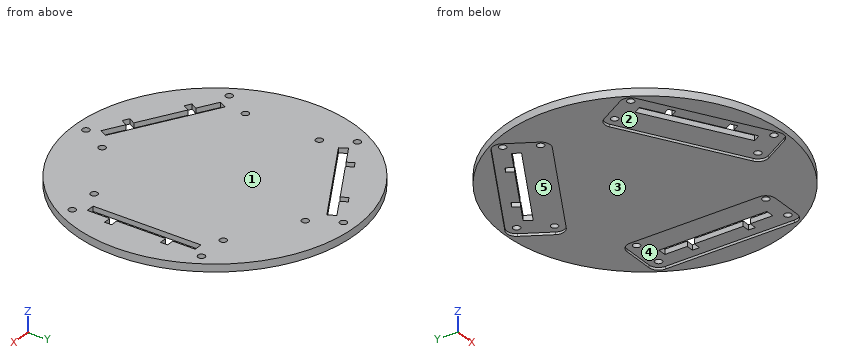
Autodesk Inventor part; units mm, degrees
ref_plane "YZ Plane" through (0, 0, 0) normal (1, 0, 0) x (0, 1, 0)
ref_plane "XZ Plane" through (0, 0, 0) normal (0, 1, 0) x (-1, 0, 0)
ref_plane "XY Plane" through (0, 0, 0) normal (0, 0, 1) x (1, 0, 0)
sketch "Skizze1" plane through (0, 0, 0) normal (0, 0, 1) x (1, 0, 0)
  line L0 (0, 78.2107) -> (0, -78.2107) construction
  line L1 (-128.6657, 0) -> (86.6199, 0) construction
  line L2 (31.7553, 29.05) -> (44.1553, 29.05) construction
  line L3 (47.5553, 25.65) -> (47.5553, -25.65) construction
  line L4 (44.1553, -29.05) -> (31.7553, -29.05) construction
  line L5 (28.3553, -25.65) -> (28.3553, 25.65) construction
  arc A0 (31.7553, 29.05) -> (28.3553, 25.65) centre (31.7553, 25.65) ccw construction
  arc A1 (47.5553, 25.65) -> (44.1553, 29.05) centre (44.1553, 25.65) ccw construction
  arc A2 (44.1553, -29.05) -> (47.5553, -25.65) centre (44.1553, -25.65) ccw construction
  arc A3 (28.3553, -25.65) -> (31.7553, -29.05) centre (31.7553, -25.65) ccw construction
  circle A4 centre (31.7553, 25.65) radius 1.4
  circle A5 centre (44.1553, 25.65) radius 1.4
  circle A6 centre (31.7553, -25.65) radius 1.4
  circle A7 centre (44.1553, -25.65) radius 1.4
  line L6 (41.6553, 21.4) -> (41.6553, -21.4)
  line L7 (38.3553, 21.4) -> (38.3553, -21.4)
  line L8 (38.3553, 21.4) -> (41.6553, 21.4)
  line L9 (38.3553, -21.4) -> (41.6553, -21.4)
  line L10 (38.3553, 0.8) -> (41.6553, 0.8)
  line L11 (38.3553, -0.8) -> (41.6553, -0.8)
  line L12 (41.6553, 12.5) -> (44.5713, 12.5)
  line L13 (44.5713, 12.5) -> (44.5713, 9.7)
  line L14 (44.5713, 9.7) -> (41.6553, 9.7)
  line L15 (41.6553, -9.7) -> (44.5713, -9.7)
  line L16 (44.5713, -9.7) -> (44.5713, -12.5)
  line L17 (44.5713, -12.5) -> (41.6553, -12.5)
  line L18 (44.1553, 29.45) -> (31.7553, 29.45)
  arc A8 (31.7553, 29.45) -> (27.9553, 25.65) centre (31.7553, 25.65) ccw
  line L19 (27.9553, 25.65) -> (27.9553, -25.65)
  arc A9 (27.9553, -25.65) -> (31.7553, -29.45) centre (31.7553, -25.65) ccw
  line L20 (31.7553, -29.45) -> (44.1553, -29.45)
  arc A10 (44.1553, -29.45) -> (47.9553, -25.65) centre (44.1553, -25.65) ccw
  line L21 (47.9553, -25.65) -> (47.9553, 25.65)
  arc A11 (47.9553, 25.65) -> (44.1553, 29.45) centre (44.1553, 25.65) ccw
  line L22 (25.9072, -29.1198) -> (28.4872, -27.589) construction
  line L23 (-0.6447, 43.9167) -> (-2.2947, 46.7745)
  circle A12 centre (0.1359, 51.0646) radius 1.4
  arc A13 (3.0804, 52.7646) -> (-1.5641, 54.0091) centre (0.1359, 51.0646) ccw construction
  arc A14 (3.4268, 52.9646) -> (-1.7641, 54.3555) centre (0.1359, 51.0646) ccw
  circle A15 centre (6.3359, 40.3259) radius 1.4
  line L24 (12.2649, 36.9962) -> (9.6492, 38.4652) construction
  arc A16 (8.0359, 37.3814) -> (9.2804, 42.0259) centre (6.3359, 40.3259) ccw construction
  arc A17 (8.2359, 37.035) -> (9.6268, 42.2259) centre (6.3359, 40.3259) ccw
  line L25 (9.6268, 42.2259) -> (3.4268, 52.9646)
  line L26 (3.0804, 52.7646) -> (9.2804, 42.0259) construction
  line L27 (-41.0357, 12.9759) -> (-47.2357, 23.7146) construction
  arc A18 (-41.0357, 12.9759) -> (-36.3912, 11.7314) centre (-38.0912, 14.6759) ccw construction
  circle A19 centre (-38.0912, 14.6759) radius 1.4
  circle A20 centre (-44.2912, 25.4146) radius 1.4
  arc A21 (-41.3821, 12.7759) -> (-36.1912, 11.385) centre (-38.0912, 14.6759) ccw
  line L28 (-47.5821, 23.5146) -> (-41.3821, 12.7759)
  arc A22 (-45.9912, 28.3591) -> (-47.2357, 23.7146) centre (-44.2912, 25.4146) ccw construction
  arc A23 (-46.1912, 28.7055) -> (-47.5821, 23.5146) centre (-44.2912, 25.4146) ccw
  line L29 (-11.4603, 44.8499) -> (-10.0023, 42.3245)
  line L30 (-13.8852, 43.4499) -> (-11.4603, 44.8499)
  line L31 (-12.4272, 40.9245) -> (-13.8852, 43.4499)
  line L32 (-37.7106, 22.5167) -> (-39.3606, 25.3745)
  line L33 (-31.653, 29.8245) -> (-33.111, 32.3499)
  line L34 (-33.111, 32.3499) -> (-30.6861, 33.7499)
  line L35 (-30.6861, 33.7499) -> (-29.2281, 31.2245)
  line L36 (-19.8705, 32.8167) -> (-21.5205, 35.6745)
  line L37 (-18.4848, 33.6167) -> (-20.1348, 36.4745)
  line L38 (-39.3606, 25.3745) -> (-2.2947, 46.7745)
  line L39 (-1.7641, 54.3555) -> (-46.1912, 28.7055)
  line L40 (-45.9912, 28.3591) -> (-1.5641, 54.0091) construction
  line L41 (8.0359, 37.3814) -> (-36.3912, 11.7314) construction
  line L42 (-36.1912, 11.385) -> (8.2359, 37.035)
  line L43 (-37.7106, 22.5167) -> (-0.6447, 43.9167)
  line L44 (-37.7106, -22.5167) -> (-39.3606, -25.3745)
  circle A24 centre (-44.2912, -25.4146) radius 1.4
  arc A25 (-47.2357, -23.7146) -> (-45.9912, -28.3591) centre (-44.2912, -25.4146) ccw construction
  arc A26 (-47.5821, -23.5146) -> (-46.1912, -28.7055) centre (-44.2912, -25.4146) ccw
  circle A27 centre (-38.0912, -14.6759) radius 1.4
  line L45 (-38.1721, -7.8764) -> (-38.1364, -10.8762) construction
  arc A28 (-36.3912, -11.7314) -> (-41.0357, -12.9759) centre (-38.0912, -14.6759) ccw construction
  arc A29 (-36.1912, -11.385) -> (-41.3821, -12.7759) centre (-38.0912, -14.6759) ccw
  line L46 (-41.3821, -12.7759) -> (-47.5821, -23.5146)
  line L47 (-47.2357, -23.7146) -> (-41.0357, -12.9759) construction
  line L48 (9.2804, -42.0259) -> (3.0804, -52.7646) construction
  arc A30 (9.2804, -42.0259) -> (8.0359, -37.3814) centre (6.3359, -40.3259) ccw construction
  circle A31 centre (6.3359, -40.3259) radius 1.4
  circle A32 centre (0.1359, -51.0646) radius 1.4
  arc A33 (9.6268, -42.2259) -> (8.2359, -37.035) centre (6.3359, -40.3259) ccw
  line L49 (3.4268, -52.9646) -> (9.6268, -42.2259)
  arc A34 (-1.5641, -54.0091) -> (3.0804, -52.7646) centre (0.1359, -51.0646) ccw construction
  arc A35 (-1.7641, -54.3555) -> (3.4268, -52.9646) centre (0.1359, -51.0646) ccw
  line L50 (-33.111, -32.3499) -> (-31.653, -29.8245)
  line L51 (-30.6861, -33.7499) -> (-33.111, -32.3499)
  line L52 (-29.2281, -31.2245) -> (-30.6861, -33.7499)
  line L53 (-0.6447, -43.9167) -> (-2.2947, -46.7745)
  line L54 (-10.0023, -42.3245) -> (-11.4603, -44.8499)
  line L55 (-11.4603, -44.8499) -> (-13.8852, -43.4499)
  line L56 (-13.8852, -43.4499) -> (-12.4272, -40.9245)
  line L57 (-18.4848, -33.6167) -> (-20.1348, -36.4745)
  line L58 (-19.8705, -32.8167) -> (-21.5205, -35.6745)
  line L59 (-2.2947, -46.7745) -> (-39.3606, -25.3745)
  line L60 (-46.1912, -28.7055) -> (-1.7641, -54.3555)
  line L61 (-1.5641, -54.0091) -> (-45.9912, -28.3591) construction
  line L62 (-36.3912, -11.7314) -> (8.0359, -37.3814) construction
  line L63 (8.2359, -37.035) -> (-36.1912, -11.385)
  line L64 (-0.6447, -43.9167) -> (-37.7106, -22.5167)
  line L65 (-31.8985, 33.0499) -> (-43.6029, 53.3224) construction
  line L66 (-34.0905, 36.8465) -> (-97.9106, 0) construction
  line L67 (-31.8985, -33.0499) -> (-43.7977, -53.6598) construction
  line L68 (-34.0905, -36.8465) -> (-97.9106, 0) construction
  circle A36 centre (0, 0) radius 55.8648
  line L69 (-48.4545, 27.8035) -> (-47.5871, 27.3058) construction
  line L70 (-42.3106, 30.4841) -> (-24.7106, 0) construction
  dimension "d1" = 58.1
  dimension "d2" = 19.2
  dimension "d3" = 3.4
  dimension "d5" = 2.8
  dimension "d6" = 5.9
  dimension "d7" = 3.3
  dimension "d8" = 20.6
  dimension "d9" = 1.6
  dimension "d10" = 2.984
  dimension "d11" = 2.8
  dimension "d12" = 19.4
  dimension "d21" = 0.4
  dimension "d22" = 3
  dimension "d32" = 360
  dimension "d44" = 1
  dimension "d45" = 1
  dimension "d47" = 1
  dimension "d53" = 35.2
extrude "Extrusion5" add sketch "Skizze1" along normal blind 3 contours A11 L21 A10 L20 A9 L19 A8 L18 | L25 A17 L42 A21 L28 A23 L39 A14 | L46 A29 L63 A33 L49 A35 L60 A26 | A36
extrude "Extrusion4" cut sketch "Skizze1" along normal blind 1 contours L10 L6 L11 L7 | A11 L21 A10 L20 A9 L19 A8 L18 | L43 L36 L38 L37 | L25 A17 L42 A21 L28 A23 L39 A14 | L64 L57 L59 L58 | L46 A29 L63 A33 L49 A35 L60 A26
equation "\"d22\" = d20"
properties part number "Stewart-Platform-Base-Innenanordnung"
Verification items for the finished model (mm, model axes). Face numbers are marked on the shaded views. A direction names the side the tool comes from. Round coordinates to 2 decimals unless told otherwise and drop trailing zeros. Loops run counter-clockwise (first coordinate to the right, second up) from the corner with the lowest first, then second, coordinate; pieces in that order, holes last. Notation, with made-up numbers: (-15.75, -20.5) - (13.25, -20.5) arc R18 cw to (13.25, 12.5) - close; hole circle Ø8 at (-13, -14.75). An arc over 180 degrees is marked (long way). Use one line per item in the form item = value.
1. Section check C-C on z = 2. Give the number of separate pieces and of enclosed holes in the cut face, and give its area (3 significant figures).
A:
separate_pieces = 1
enclosed_holes = 15
area = 9,260 mm²
2. Draft check along Y on the marked faces 3, 4 and 5. Enter one of: pulls with the +Y half, pulls with the -Y half, needs draft (parallel to the pull), parting line crosses it, or undercut.
A:
face_3 = needs draft
face_4 = undercut
face_5 = undercut
3. Gauge pin test, flat ends, axial feed: pin 1 Ø1.6 at (x, z) = (43, 2) entering from -Y; pin 2 Ø1.5 at (y, z) = (-38, 0.5) entering from +X; pin 3 Ø1 at (x, z) = (43.5, 2.5) entering from +Y; pin 4 Ø2 at (x, y) = (0.14, -51.06) entering from +Z. Record the tip position at first contact, or that the pin passes through.
A:
pin_1 = -36.61
pin_2 = 41.63
pin_3 = 35.66
pin_4 = through
4. Section check B-B on y = -19. Record the cut outline in (x, z), and give its area (3 significant figures).
A:
outline = (-52.53, 0) - (-44.98, 0) - (-44.98, 1) - (-23, 1) - (-23, 0) - (27.96, 0) - (27.96, 1) - (38.36, 1) - (38.36, 3) - (-52.53, 3) - close; (41.66, 1) - (47.96, 1) - (47.96, 0) - (52.53, 0) - (52.53, 3) - (41.66, 3) - close
area = 267 mm²
5. Scan lines: probe 1 along Y at (x, z) = (-45, 1.8); probe 2 along X at (y, z) = (13, 1.25); probe 3 along Y at (x, z) = (-20, 2.5). Record each from-to range of solid material in increasing order.
A:
probe_1 = -33.1 to -26.62, -24.21 to 24.21, 26.62 to 33.1
probe_2 = -54.33 to 38.36, 41.66 to 54.33
probe_3 = -52.16 to -36.55, -32.74 to 32.74, 36.55 to 52.16
6. Access from +Z, -Z, +X, -X, +Y, -Y to the whole of each face (thin tool, end or side, straight path). Record for the marked faces 1 and 2.
A:
face_1 = +Z, +X, -X, +Y, -Y
face_2 = -Z
7. Section check A-A on y = 0. Record the cut outline in (x, z), and give its area (3 significant figures).
A:
outline = (-55.86, 0) - (27.96, 0) - (27.96, 1) - (38.36, 1) - (38.36, 3) - (-55.86, 3) - close; (41.66, 1) - (47.96, 1) - (47.96, 0) - (55.86, 0) - (55.86, 3) - (41.66, 3) - close
area = 309 mm²
